Verification items for the finished model (mm, model axes). Face numbers are marked on the shaded views. A direction names the side the tool comes from. Coordinates: 2 decimals unless noted, no trailing zeros. Write each loop counter-clockwise with the first axis right and the second up, starting at its lowest first coordinate (ties: lowest second). Pieces come first, ordered by that corner, then holes. Notation, with made-up numbers: M 80,-14.5 L 118,-14.5 A24 cw 118,6.5 Z; hole C 45.5,-2.75 d1. An arc over 180 degrees is marked long. One line per item, written item: value.
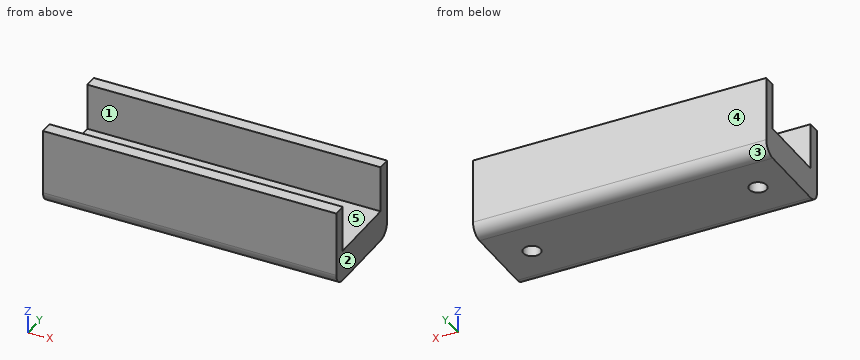
```python
from build123d import *

# Parameters (mm, degrees)
SKETCH1_W           = 60
SKETCH1_H           = 20
SKETCH1_R           = 1.75
BOSS_EXTRUDE1_DEPTH = 6.35
SKETCH2_W           = 60
SKETCH2_H           = 2.54
BOSS_EXTRUDE2_DEPTH = 9.525
FILLET1_R           = 2.54


with BuildPart() as part:
    # Sketch1 → Boss-Extrude1 (new body)
    with BuildSketch(Plane.XY):
        Rectangle(SKETCH1_W, SKETCH1_H)
        with Locations((-23.12, 0)):
            Circle(SKETCH1_R, mode=Mode.SUBTRACT)
        with Locations((23.12, 0)):
            Circle(SKETCH1_R, mode=Mode.SUBTRACT)
    extrude(amount=BOSS_EXTRUDE1_DEPTH)

    # Sketch2 → Boss-Extrude2 (add)
    with BuildSketch(Plane.XY.offset(6.35)):
        with Locations((0, 8.73)):
            Rectangle(SKETCH2_W, SKETCH2_H)
        with Locations((0, -8.73)):
            Rectangle(SKETCH2_W, SKETCH2_H)
    extrude(amount=BOSS_EXTRUDE2_DEPTH)

    # Fillet1
    fillet1_edges = [part.edges().sort_by_distance(p)[0] for p in [
        (0, 10, 0),
        (0, -10, 0),
    ]]
    fillet(fillet1_edges, radius=FILLET1_R)


solid = part.part
```
Item 1: Draft check along Y on the marked faces 1, 2 and 3. Enter one of: released by +Y, released by -Y, zero draft, split by the parting line, or undercut.
The answers:
face 1: undercut
face 2: zero draft
face 3: released by +Y
Item 2: Cross-section at B-B, the plane x = -23.12. Enter the section's corners in (y, z) (3 decimals).
The answers:
outline: M -10,2.54 A2.54 ccw -7.46,0 L -1.75,0 L -1.75,6.35 L -7.46,6.35 L -7.46,15.875 L -10,15.875 Z; M 1.75,0 L 7.46,0 A2.54 ccw 10,2.54 L 10,15.875 L 7.46,15.875 L 7.46,6.35 L 1.75,6.35 Z
Item 3: Cross-section at D-D, the plane x = -17. Enter the section's corners in (y, z) (3 decimals), and give its area (3 significant figures).
The answers:
outline: M -10,2.54 A2.54 ccw -7.46,0 L 7.46,0 A2.54 ccw 10,2.54 L 10,15.875 L 7.46,15.875 L 7.46,6.35 L -7.46,6.35 L -7.46,15.875 L -10,15.875 Z
area: 173 mm²
Item 4: Go/stop test with a flat-tipped pin: P1, Ø4.5, axis at x = 14.5, y = -2, coming from the +Z side. Record where the tip stops, or that it passes through.
The answers:
P1: stops at z = 6.35
Item 5: Access from +Z, -Z, +X, -X, +Y, -Y to the whole of each face (thin tool, end or side, straight path). Record for the marked faces 4 and 5.
The answers:
face 4: +Z, -Z, +X, -X, +Y
face 5: +Z, +X, -X
Item 6: Cross-section at A-A, the plane y = 0. Enter the section's corners in (x, z).
The answers:
outline: M -30,0 L -24.87,0 L -24.87,6.35 L -30,6.35 Z; M -21.37,0 L 21.37,0 L 21.37,6.35 L -21.37,6.35 Z; M 24.87,0 L 30,0 L 30,6.35 L 24.87,6.35 Z
Item 7: Scan lines: line 1 (Y direction, x = 14.5, z = 11); line 2 (Y direction, x = -23.12, z = 4.25); line 3 (Z direction, x = -15, y = 2.75). Record each from-to range of solid material in increasing order.
The answers:
line 1: y = -10 to -7.46, 7.46 to 10
line 2: y = -10 to -1.75, 1.75 to 10
line 3: z = 0 to 6.35
Item 8: Cross-section at C-C, the plane z = 15. Enter the section's corners in (x, y), and give its area (3 significant figures).
The answers:
outline: M -30,-10 L 30,-10 L 30,-7.46 L -30,-7.46 Z; M -30,7.46 L 30,7.46 L 30,10 L -30,10 Z
area: 305 mm²
